For this review, use the dimensioned drawing (mm, ordinates from the lowest corner) and the shaded views. A direction names the side the tool comes from. Coordinates: 2 decimals unless noted, no trailing zeros. Order: outer loops, then holes, each group sorted by start corner. A loop starts at its lowest first (then second) coordinate and runs counter-clockwise, first axis right, second up. Notation, with made-up numbers: M -38.75,40.25 L -22.75,40.25 A28 ccw -22.75,64.25 Z; hole C -17,64.5 d5. An arc over 180 degrees is marked long. Answer in a Markdown table with one row per item.
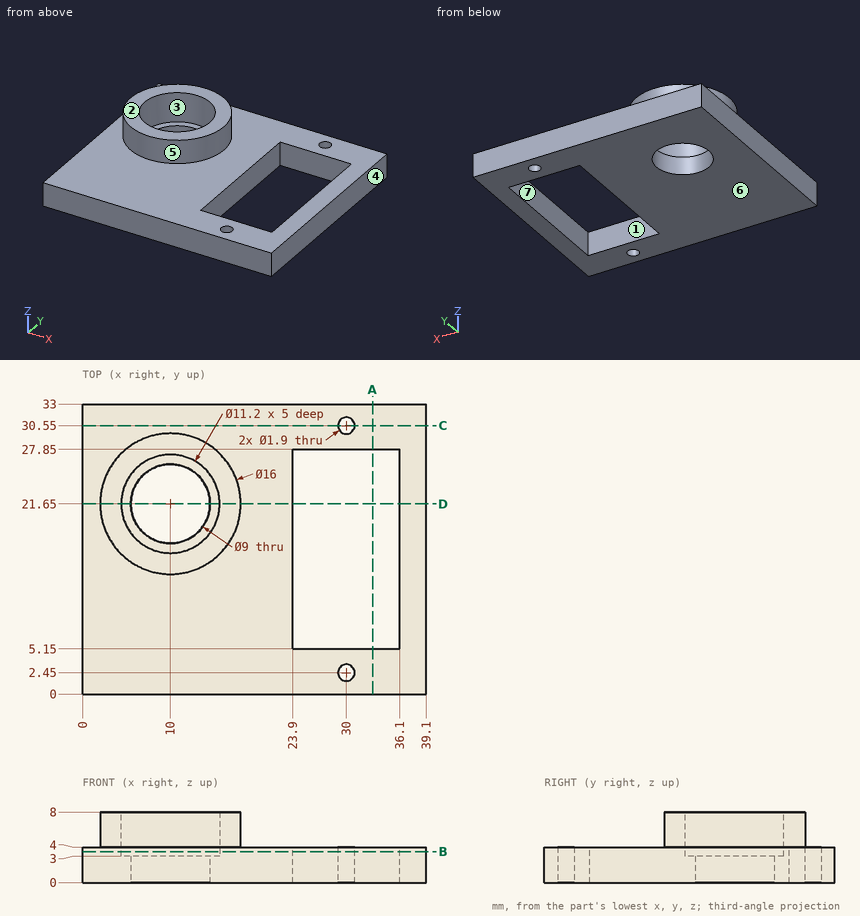
(1) Add section A-A, the plane x = 33. Give the boundary of the cut face in (y, z), and give its area (3 significant figures).
Return value:
| item | result |
|---|---|
| outline | M 0,0 L 5.15,0 L 5.15,4 L 0,4 Z; M 27.85,0 L 33,0 L 33,4 L 27.85,4 Z |
| area | 41.2 mm2 |
(2) Draft analysis for pull direction X (two halves, no side actions). For the marked faces 1, 2, 3 and 4, state which applies: pulls with the +X half, pulls with the -X half, needs draft (parallel to the pull), parting line crosses it, or undercut.
Return value:
| item | result |
|---|---|
| face 1 | undercut |
| face 2 | needs draft |
| face 3 | undercut |
| face 4 | pulls with the +X half |
(3) Add section B-B, the plane z = 3.5. Give the boundary of the cut face in (x, y).
Return value:
| item | result |
|---|---|
| outline | M 0,0 L 39.1,0 L 39.1,33 L 0,33 Z; hole C 10,21.65 d11.2; hole M 23.9,5.15 L 36.1,5.15 L 36.1,27.85 L 23.9,27.85 Z; hole C 30,2.45 d1.9; hole C 30,30.55 d1.9 |
(4) Insertion check: pin 1 Ø1.7 at (x, y) = (30, 30.55) entering from +Z; pin 2 Ø16.5 at (x, y) = (25.5, 12) entering from +Z. Each pin has a flat end and moves straight along its axis. Give the tip position at first contact, or say it passes through.
Return value:
| item | result |
|---|---|
| pin 1 | passes through |
| pin 2 | stops at z = 4 |
(5) Add section C-C, the plane y = 30.55. Give the boundary of the cut face in (x, z), and give its area (3 significant figures).
Return value:
| item | result |
|---|---|
| outline | M 0,0 L 29.05,0 L 29.05,4 L 0,4 Z; M 30.95,0 L 39.1,0 L 39.1,4 L 30.95,4 Z |
| area | 149 mm2 |
(6) For line 1 along Y through (x, z) = (30, 2.6); line 2 along Y through (x, z) = (28.5, 3.25); line 3 along Y through (x, z) = (10, 1.6), list the stretches that pass through material, from the lowest coordinate up. Write a range as from..to.
Return value:
| item | result |
|---|---|
| line 1 | y = 0..1.5, 3.4..5.15, 27.85..29.6, 31.5..33 |
| line 2 | y = 0..5.15, 27.85..33 |
| line 3 | y = 0..17.15, 26.15..33 |
(7) Add section D-D, the plane y = 21.65. Give the boundary of the cut face in (x, z).
Return value:
| item | result |
|---|---|
| outline | M 0,0 L 5.5,0 L 5.5,3 L 4.4,3 L 4.4,8 L 2,8 L 2,4 L 0,4 Z; M 14.5,0 L 23.9,0 L 23.9,4 L 18,4 L 18,8 L 15.6,8 L 15.6,3 L 14.5,3 Z; M 36.1,0 L 39.1,0 L 39.1,4 L 36.1,4 Z |
(8) For the marked faces 5, 6 and 7, list the 3-axis set-ups (+Z, -Z, +X, -X, +Y, -Y) from which the entire face can be reached by the end or side of a thin tool; tool diameter is ignored.
Return value:
| item | result |
|---|---|
| face 5 | +Z |
| face 6 | -Z, +X, -X, +Y, -Y |
| face 7 | +Z, -Z |
